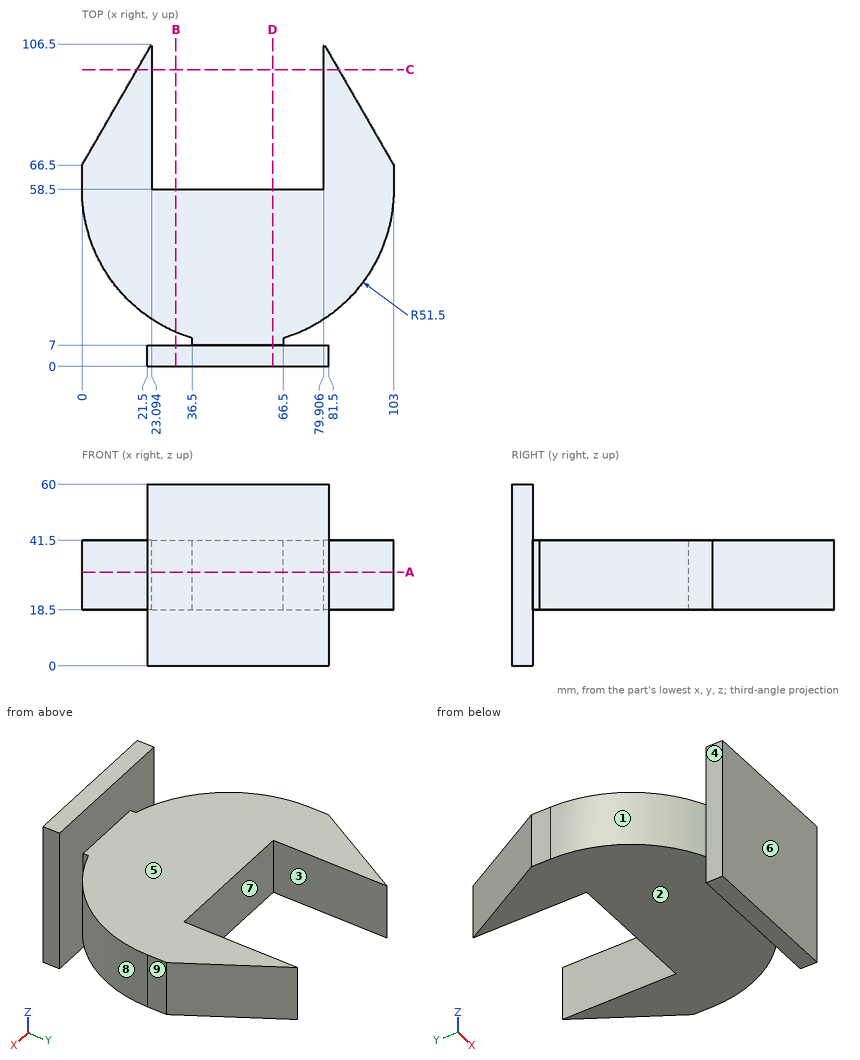
Study the drawing (mm; zero at the part's minimum x, y, z) and answer. A direction names the side the tool comes from. Round coordinates to 2 decimals unless told otherwise and drop trailing zeros. Write each loop counter-clockwise with the first axis right and the second up, starting at its lowest first coordinate (ties: lowest second). Pieces come first, ordered by that corner, then holes. Notation, with made-up numbers: (16, 89) - (71, 89) arc R16 ccw to (71, 111) - close; hole circle Ø1 at (26.25, 29.5). An arc over 180 degrees is marked (long way). Use a Markdown table: item, result. Add a question column.
1. The part is cut by section C-C (y = 98). Write down the section's boundary in (x, z).
2. The part is cut by section B-B (x = 31). Write down the section's boundary in (y, z).
3. Consider line 1 (X direction, y = 61, z = 19); line 2 (Y direction, x = 63, z = 5.5); line 3 (Z direction, x = 15, y = 26). Determine where each line is inside the solid, lowest interval first.
4. Flat-ended cylindrical pins translate along their axes: P1, Ø3.5, axis at y = 4.5, z = 43, coming from the -X side; P2, Ø5.5, axis at y = 3.5, z = 20, coming from the +X side; P3, Ø8, axis at x = 25, y = 40, coming from the -Z side. Find the tip coordinate at first contact, or state that the pin passes through.
5. For a pull along Y with two mould halves and no side action, classify the marked faces 6, 7, 8 and 9 as +Y half, -Y half, draft (parallel to the pull), parting line (faces both ways), or undercut.
6. The part is cut by section D-D (x = 63). Write down the section's boundary in (y, z).
7. The part is cut by section A-A (z = 31). Write down the section's boundary in (x, y), and give its area (3 significant figures).
8. A tool of negligible diameter and unlimited length cuts with its end or side. For the marked faces 1, 2, 3, 4 and 5, from which of +Z, -Z, +X, -X, +Y, -Y can it reach the whole face along a straight path? Write none if from no direction.
Reported:
| question | item | result |
|---|---|---|
| 1 | outline | (18.19, 18.5) - (23.09, 18.5) - (23.09, 41.5) - (18.19, 41.5) - close; (79.91, 18.5) - (84.81, 18.5) - (84.81, 41.5) - (79.91, 41.5) - close |
| 2 | outline | (0, 0) - (7, 0) - (7, 60) - (0, 60) - close; (11.26, 18.5) - (58.5, 18.5) - (58.5, 41.5) - (11.26, 41.5) - close |
| 3 | line 1 | 0 to 23.09, 79.91 to 103 |
| 3 | line 2 | 0 to 7 |
| 3 | line 3 | 18.5 to 41.5 |
| 4 | P1 | x = 21.5 |
| 4 | P2 | x = 81.5 |
| 4 | P3 | z = 18.5 |
| 5 | face 6 | -Y half |
| 5 | face 7 | +Y half |
| 5 | face 8 | undercut |
| 5 | face 9 | draft |
| 6 | outline | (0, 0) - (7, 0) - (7, 18.5) - (58.5, 18.5) - (58.5, 41.5) - (7, 41.5) - (7, 60) - (0, 60) - close |
| 7 | outline | (0, 58.5) arc R51.5 ccw to (36.5, 9.23) - (36.5, 7) - (21.5, 7) - (21.5, 0) - (81.5, 0) - (81.5, 7) - (66.5, 7) - (66.5, 9.23) arc R51.5 ccw to (103, 58.5) - (103, 66.5) - (79.91, 106.5) - (79.91, 58.5) - (23.09, 58.5) - (23.09, 106.5) - (0, 66.5) - close |
| 7 | area | 5,900 mm^2 |
| 8 | face 1 | +Z, -Z, -X |
| 8 | face 2 | -Z, +X, -X, +Y |
| 8 | face 3 | +Z, -Z, +Y |
| 8 | face 4 | +Z, -Z, -X, -Y |
| 8 | face 5 | +Z, +X, -X, +Y |
